Autodesk Fusion 360 part; units mm, degrees
sketch "Sketch1" plane through (0, 0, 0) normal (0, 0, 1) x (1, 0, 0)
  line L0 (5, 0) -> (306, 0)
  line L1 (311, 5) -> (311, 200)
  line L2 (306, 205) -> (5, 205)
  line L3 (0, 200) -> (0, 5)
  circle A0 centre (30, 29) radius 17
  circle A1 centre (65.8571, 29.3) radius 17
  circle A2 centre (101.7143, 29.6) radius 17
  circle A3 centre (28, 174) radius 17
  circle A4 centre (99.7143, 176) radius 17
  circle A5 centre (63.8571, 175) radius 17
  circle A6 centre (137.5714, 29.9) radius 17
  circle A7 centre (135.5714, 177) radius 17
  circle A8 centre (173.4286, 30.1) radius 17
  circle A9 centre (209.2857, 31) radius 17
  circle A10 centre (245.1429, 32) radius 17
  circle A11 centre (281, 33) radius 17
  circle A12 centre (171.4286, 177) radius 17
  circle A13 centre (207.2857, 178) radius 17
  circle A14 centre (243.1429, 179) radius 17
  circle A15 centre (279, 180) radius 17
  arc A16 (311, 200) -> (306, 205) centre (306, 200) ccw
  arc A17 (5, 205) -> (0, 200) centre (5, 200) ccw
  arc A18 (306, 0) -> (311, 5) centre (306, 5) ccw
  arc A19 (0, 5) -> (5, 0) centre (5, 5) ccw
  dimension "d1" = 311
  dimension "d2" = 205
  dimension "d4" = 34
  dimension "d6" = 29
  dimension "d8" = 34
  dimension "d9" = 34
  dimension "d10" = 34
  dimension "d11" = 34
  dimension "d13" = 34
  dimension "d14" = 34
  dimension "d15" = 34
  dimension "d16" = 34
  dimension "d17" = 34
  dimension "d18" = 34
  dimension "d19" = 34
  dimension "d28" = 29.3
  dimension "d29" = 29.6
  dimension "d30" = 29.9
  dimension "d31" = 30.1
  dimension "d32" = 31
  dimension "d33" = 32
  dimension "d34" = 33
  dimension "d35" = 34
  dimension "d36" = 34
  dimension "d37" = 34
  dimension "d38" = 34
  dimension "d48" = 31
  dimension "d49" = 30
  dimension "d50" = 29
  dimension "d51" = 28
  dimension "d52" = 28
  dimension "d53" = 27
  dimension "d55" = 30
  dimension "d56" = 35.8571
  dimension "d57" = 35.8571
  dimension "d58" = 35.8571
  dimension "d59" = 35.8571
  dimension "d60" = 35.8571
  dimension "d61" = 35.8571
  dimension "d62" = 35.8571
  dimension "d63" = 30
  dimension "d64" = 28
  dimension "d66" = 35.8571
  dimension "d67" = 35.8571
  dimension "d68" = 35.8571
  dimension "d69" = 35.8571
  dimension "d70" = 35.8571
  dimension "d71" = 35.8571
  dimension "d72" = 32
  dimension "d73" = 26
  dimension "d74" = 25
  dimension "d75" = 35.8571
  dimension "d76" = 5
  dimension "d77" = 5
  dimension "d78" = 5
  dimension "d79" = 5
sketch "Sketch2" plane through (0, 0, 0) normal (0, 0, 1) x (1, 0, 0)
extrude "Extrude1" add sketch "Sketch1" along normal blind 3.5
extrude "Extrude2" add 1 faces at (123.0248, 122.1087, 3.5) along direction (0, 0, 1) blind 1
sketch "Sketch3" plane through (0, 0, 0) normal (0, 0, 1) x (1, 0, 0)
  line L0 (5, 0) -> (306.1184, 0)
  line L1 (311.1184, 5) -> (311.1184, 55.2879)
  line L2 (311.1184, 55.2879) -> (0, 55.2879)
  line L3 (0, 55.2879) -> (0, 5)
  line L4 (310, 148.1101) -> (0, 148.1101)
  line L5 (0, 148.1101) -> (0, 199.7882)
  line L6 (5, 204.7882) -> (305, 204.7882)
  line L7 (310, 199.7882) -> (310, 148.1101)
  arc A0 (5, 204.7882) -> (0, 199.7882) centre (5, 199.7882) ccw
  arc A1 (310, 199.7882) -> (305, 204.7882) centre (305, 199.7882) ccw
  arc A2 (0, 5) -> (5, 0) centre (5, 5) ccw
  arc A3 (306.1184, 0) -> (311.1184, 5) centre (306.1184, 5) ccw
  dimension "d84" = 5
  dimension "d85" = 5
  dimension "d86" = 5
  dimension "d87" = 5
sketch "Sketch4" plane through (0, 0, 0) normal (0, 0, 1) x (1, 0, 0)
Check sheet for the modelled part. Datum: model origin and axes. Units: mm. Give positions to 0.01 mm unless a question says otherwise; leave off trailing zeros. Loops run counter-clockwise (first coordinate to the right, second up) from the corner with the lowest first, then second, coordinate; pieces in that order, holes last. Notation, with made-up numbers: M 71,-14.5 L 94,-14.5 A31 ccw 94,9.5 Z; hole C -17,73.25 d9. An arc over 180 degrees is marked long. Use a Markdown table: item, result. Add a question column.
Q1. Sectioned sample at B-B, the plane z = 2.4. Give the number of separate pieces and of enclosed holes in the cut face, then the cut area to 3 significant figures.
Q2. Sectioned sample at D-D, the plane x = 145. Record the cut outline in (y, z), then the cut area to 3 significant figures.
Q3. Mould release check, pull along Y, two halves, no side actions. Record for faces 1 (the flat face through (153, 104, 0)), 2 (the cylindrical face through (84.73, 28.85, 2.22)): pulls with the +Y half, pulls with the -Y half, needs draft (parallel to the pull), parting line crosses it, or undercut.
Q4. Scan lines: line 1 along Y through (x, z) = (97, 3.55); line 2 along Y through (x, z) = (77.5, 1.35). Record each from-to range of solid material in increasing order. Write a range as [from, to].
Q5. Sectioned sample at A-A, the plane x = 177.5. Record the cut outline in (y, z), then the cut area to 3 significant figures.
Q6. Go/stop test with a flat-tipped pin: pin 1 (20.5 mm diameter, centred on x = 99.71, y = 176, fed in from +Z). Record where the tip stops, or that it passes through.
Verdict:
| question | item | result |
|---|---|---|
| 1 | separate pieces | 1 |
| 1 | enclosed holes | 16 |
| 1 | area | 49,200 mm^2 |
| 2 | outline | M 0,0 L 14.61,0 L 14.61,4.5 L 0,4.5 Z; M 45.19,0 L 162.85,0 L 162.85,4.5 L 45.19,4.5 Z; M 191.15,0 L 205,0 L 205,4.5 L 191.15,4.5 Z |
| 2 | area | 658 mm^2 |
| 3 | face 1 | needs draft |
| 3 | face 2 | undercut |
| 4 | line 1 | [0, 13.27], [45.93, 159.22], [192.78, 205] |
| 4 | line 2 | [0, 16.91], [41.69, 164.86], [185.14, 205] |
| 5 | outline | M 0,0 L 13.59,0 L 13.59,4.5 L 0,4.5 Z; M 46.61,0 L 161.12,0 L 161.12,4.5 L 46.61,4.5 Z; M 192.88,0 L 205,0 L 205,4.5 L 192.88,4.5 Z |
| 5 | area | 631 mm^2 |
| 6 | pin 1 | through |
